Check sheet for the modelled part. Datum: model origin and axes. Units: mm. Coordinates: 2 decimals unless noted, no trailing zeros. Order: outer loops, then holes, each group sorted by start corner. A loop starts at its lowest first (then second) coordinate and runs counter-clockwise, first axis right, second up.
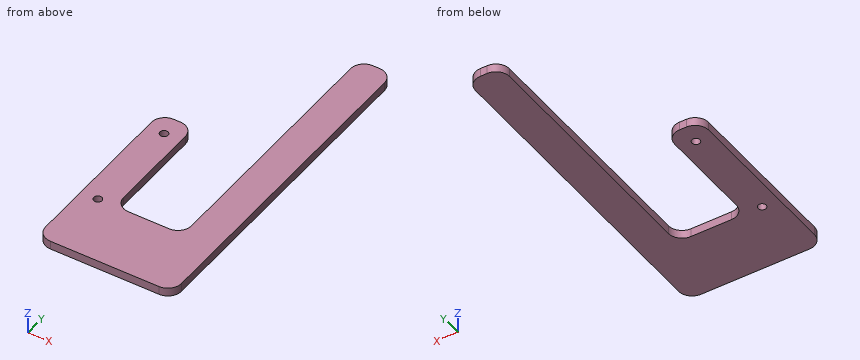
from build123d import *

# Parameters (mm, degrees)
F0_R     = 1.524
F0_W     = 12.7
F0_H     = 25.4
F1_DEPTH = 3.175
F2_R     = 5.08


with BuildPart() as f1:
    # F0 (on Top) → F1 (new body)
    with BuildSketch(Plane.XY):
        Polygon((1.1870916933, -2.6605168543), (-24.2129083067, -2.6605168543), (-24.2129083067, 42.9525971413), (-36.9129083067, 42.9525971413), (-36.9129083067, -2.6605168543), (-36.9129083067, -12.0184096301), (-36.9129083067, -28.0605168543), (13.8870916933, -28.0605168543), (13.8870916933, -12.0184096301), (13.8870916933, -2.6605168543), (13.8870916933, 73.5394831457), (1.1870916933, 73.5394831457), align=None)
        with Locations((-30.5629083067, -2.6605168543)):
            Circle(F0_R, mode=Mode.SUBTRACT)
        with Locations((-30.5629083067, 35.4394831457)):
            Circle(F0_R, mode=Mode.SUBTRACT)
        with Locations((7.5370916933, 86.2394831457)):
            Rectangle(F0_W, F0_H)
    extrude(amount=F1_DEPTH)

    # F2
    f2_edges = [f1.edges().sort_by_distance(p)[0] for p in [
        (-36.912908, 42.952597, 1.5875),
        (1.187092, -2.660517, 1.5875),
        (-36.912908, -28.060517, 1.5875),
        (13.887092, -28.060517, 1.5875),
        (-24.212908, -2.660517, 1.5875),
        (1.187092, 98.939483, 1.5875),
        (13.887092, 98.939483, 1.5875),
        (-24.212908, 42.952597, 1.5875),
    ]]
    fillet(f2_edges, radius=F2_R)


solid = f1.part
(1) Cross-section at A-A (y = 12.5). Enter the section's corners in (x, z) (3 decimals), and give its area (3 significant figures).
Filled in:
outline: (-36.913, 0) - (-24.213, 0) - (-24.213, 3.175) - (-36.913, 3.175) - close; (1.187, 0) - (13.887, 0) - (13.887, 3.175) - (1.187, 3.175) - close
area: 80.6 mm2
(2) Cross-section at B-B (z = 0.5). Enter the section's corners in (x, y).
Filled in:
outline: (-36.91, -22.98) arc R5.08 ccw to (-31.83, -28.06) - (8.81, -28.06) arc R5.08 ccw to (13.89, -22.98) - (13.89, 93.86) arc R5.08 ccw to (8.81, 98.94) - (6.27, 98.94) arc R5.08 ccw to (1.19, 93.86) - (1.19, 2.42) arc R5.08 cw to (-3.89, -2.66) - (-19.13, -2.66) arc R5.08 cw to (-24.21, 2.42) - (-24.21, 37.87) arc R5.08 ccw to (-29.29, 42.95) - (-31.83, 42.95) arc R5.08 ccw to (-36.91, 37.87) - close; hole circle Ø3.05 at (-30.56, -2.66); hole circle Ø3.05 at (-30.56, 35.44)
(3) Cross-section at D-D (y = 41.5). Enter the section's corners in (x, z) (3 decimals).
Filled in:
outline: (-35.389, 0) - (-25.736, 0) - (-25.736, 3.175) - (-35.389, 3.175) - close; (1.187, 0) - (13.887, 0) - (13.887, 3.175) - (1.187, 3.175) - close
(4) Go/stop test with flat-tipped pins: P1, Ø1.6, axis at x = -14.5, z = 1, coming from the +Y side; P2, Ø5, axis at x = -3.5, y = 26, coming from the -Z side; P3, Ø0.8, axis at x = -31, z = 1.5, coming from the +Y side; P4, Ø3.5, axis at x = -30.56, y = -2.66, coming from the -Z side. Record where each tip stops, or that it passes through.
Filled in:
P1: stops at y = -2.66
P2: passes through
P3: stops at y = 42.95
P4: stops at z = 0
(5) Cross-section at C-C (x = -6.5). Enter the section's corners in (y, z) (3 decimals), and give its area (3 significant figures).
Filled in:
outline: (-28.061, 0) - (-2.661, 0) - (-2.661, 3.175) - (-28.061, 3.175) - close
area: 80.6 mm2
(6) Thickness scan on probe 1 along Y at (x, z) = (-30, 0.25); probe 2 along X at (y, z) = (21, 1.2); probe 3 along X at (y, z) = (66, 1.7). Record the ranges inside material, lowest first.
Filled in:
probe 1: y = -28.06 to -4.08, -1.24 to 34.02, 36.86 to 42.95
probe 2: x = -36.91 to -24.21, 1.19 to 13.89
probe 3: x = 1.19 to 13.89
